Autodesk Inventor part; units mm, degrees
ref_plane "YZ Plane" through (0, 0, 0) normal (1, 0, 0) x (0, 1, 0)
ref_plane "XZ Plane" through (0, 0, 0) normal (0, 1, 0) x (-1, 0, 0)
ref_plane "XY Plane" through (0, 0, 0) normal (0, 0, 1) x (1, 0, 0)
sketch "Sketch1" plane through (0, 0, 0) normal (0, 0, 1) x (1, 0, 0)
  line L0 (-25, 10) -> (10, 10)
  line L1 (10, 10) -> (10, -10)
  line L2 (10, -10) -> (-25, -10)
  line L3 (-25, 5) -> (-20, 5)
  line L4 (-20, 5) -> (-20, -5)
  line L5 (-20, -5) -> (-25, -5)
  line L6 (-25, -10) -> (-25, -5)
  line L7 (-25, 5) -> (-25, 10)
  circle A0 centre (0, 0) radius 2.5
  point P0 (10, 0)
  dimension "d0" = 5
  dimension "d1" = 10
  dimension "d2" = 5
  dimension "d3" = 5
  dimension "d4" = 5
  dimension "d5" = 35
  dimension "d7" = 10
  dimension "d8" = 5
extrude "Extrusion1" add sketch "Sketch1" along normal blind 10
sketch "Sketch2" plane through (0, 0, 10) normal (0, 0, 1) x (1, 0, 0)
  circle A0 centre (0, 0) radius 2.5
  circle A1 centre (0, 0) radius 5
  dimension "d11" = 10
extrude "Extrusion2" cut sketch "Sketch2" against normal blind 2
equation "\"BendRadius\" = Thickness"
equation "\"BendReliefWidth\" = Thickness"
equation "\"BendReliefDepth\" = 0.5 * Thickness"
equation "\"CornerReliefSize\" = 4 * Thickness"
equation "\"MinimumRemnant\" = 2 * Thickness"
equation "\"TransitionRadius\" = BendRadius"
equation "\"JacobiRadiusSize\" = BendRadius"
equation "\"GapSize\" = Thickness"
properties part number "lesson1"
Design review of the part built by this model. Coordinates are the model's own, in mm. A direction names the side the tool comes from. Give positions to 0.01 mm unless a question says otherwise; leave off trailing zeros. Order: outer loops, then holes, each group sorted by start corner. A loop starts at its lowest first (then second) coordinate and runs counter-clockwise, first axis right, second up. Notation, with made-up numbers: (-13.5, 80) -> (15.5, 80) arc R5 ccw to (15.5, 87) -> close; hole circle Ø10 at (60.5, -2.75). An arc over 180 degrees is marked (long way). Write item = value, one per line. Start each with the question number.
(1) For pin 1 (1 mm diameter, centred on x = 3.5, y = 4.5, fed in from -Z); pin 2 (9 mm diameter, centred on x = 0, y = 0, fed in from +Z); pin 3 (2 mm diameter, centred on y = -2, z = 7.5, fed in from -X), all flat-tipped, find the tip position at first contact; note any pin that passes through.
(2) We need section C-C on x = 0. Write out the cut boundary in (y, z).
(3) Mouldability with a two-part tool opening along Y and no side actions: class faces 4 (the face through (-8, 10, 5)), 5 (the face through (10, 0, 5)), 6 (the face through (2, -2, 8)), 7 (the face through (-7, -10, 5)) as +Y half, -Y half, draft (parallel to the pull), parting line (faces both ways), or undercut.
(4) For faces 1 (the face through (-1.08, -4.88, 9.01)), 2 (the face through (-8, 0, 0)), 3 (the face through (-20, 0, 5)), list the 3-axis set-ups (+Z, -Z, +X, -X, +Y, -Y) from which the entire face can be reached by the end or side of a thin tool; tool diameter is ignored.
(5) We need section B-B on z = 1.75. Write out the cut boundary in (x, y).
(6) To check wall thickness, follow line 1 along Y through (x, z) = (0, 6.25); line 2 along Y through (x, z) = (0, 9.4); line 3 along X through (y, z) = (-3.25, 1.5). State the ranges of each line that lie inside material, in increasing order.
(7) We need section A-A on y = 0. Write out the cut boundary in (x, z).
Numbers:
q1.pin_1 = 0
q1.pin_2 = 8
q1.pin_3 = -20
q2.outline = (-10, 0) -> (-2.5, 0) -> (-2.5, 8) -> (-5, 8) -> (-5, 10) -> (-10, 10) -> close; (2.5, 0) -> (10, 0) -> (10, 10) -> (5, 10) -> (5, 8) -> (2.5, 8) -> close
q3.face_4 = +Y half
q3.face_5 = draft
q3.face_6 = undercut
q3.face_7 = -Y half
q4.face_1 = +Z
q4.face_2 = -Z, +X, -X, +Y, -Y
q4.face_3 = +Z, -Z, -X
q5.outline = (-25, -10) -> (10, -10) -> (10, 10) -> (-25, 10) -> (-25, 5) -> (-20, 5) -> (-20, -5) -> (-25, -5) -> close; hole circle Ø5 at (0, 0)
q6.line_1 = -10 to -2.5, 2.5 to 10
q6.line_2 = -10 to -5, 5 to 10
q6.line_3 = -20 to 10
q7.outline = (-20, 0) -> (-2.5, 0) -> (-2.5, 8) -> (-5, 8) -> (-5, 10) -> (-20, 10) -> close; (2.5, 0) -> (10, 0) -> (10, 10) -> (5, 10) -> (5, 8) -> (2.5, 8) -> close
